from build123d import *

# Parameters (mm, degrees)
F0_R     = 25
F1_DEPTH = 5
F2_R     = 10
F3_DEPTH = 70
F4_R     = 19
F5_DEPTH = 5


with BuildPart() as f1:
    # F0 (on Front) → F1 (new body)
    with BuildSketch(Plane.XZ):
        Circle(F0_R)
    extrude(amount=F1_DEPTH)

    # F2 (on face) → F3 (join)
    with BuildSketch(Plane.XZ.offset(5)):
        Circle(F2_R)
    extrude(amount=F3_DEPTH)

    # F4 (on face) → F5 (join)
    with BuildSketch(Plane.XZ.offset(75)):
        Circle(F4_R)
    extrude(amount=F5_DEPTH)


solid = f1.part
Part model, mm, in its own coordinate system. A direction names the side the tool comes from. Coordinates: 2 decimals unless noted, no trailing zeros. Loops run counter-clockwise (first coordinate to the right, second up) from the corner with the lowest first, then second, coordinate; pieces in that order, holes last. Notation, with made-up numbers: (76, -15) - (86, -15) arc R8 cw to (86, -5) - close; hole circle Ø4 at (86.25, -37). An arc over 180 degrees is marked (long way). Write each question's results on one line, items separated by ' | '. Start each with the question number.
Q1. Slice it at D-D on y = -14. Give the cut face in (x, z).
Q2. Which spindle directions (+Z, -Z, +X, -X, +Y, -Y) get a long thin tool onto all of the face, cutting with end or side? Do faces 5 (the cylindrical face through (-2.17, -39.51, -9.76)), 6 (the cylindrical face through (8.767, -77.465, -16.856)), 7 (the cylindrical face through (23.846, -2.465, 7.509)). Say none if no direction does.
Q3. Drop flat-ended pins along their axis: pin 1 Ø3 at (y, z) = (-25.5, 5) entering from -X; pin 2 Ø12 at (x, y) = (11.5, -18) entering from +Z; pin 3 Ø5 at (y, z) = (-64, -9.5) entering from +X. Give the stop position or say it passes through.
Q4. Slice it at B-B on x = 0. Give the cut face in (y, z).
Q5. Two-plate mould, pull along Y, no slides. Class faces 1 (the flat face through (0, 0, 0)), 2 (the flat face through (0, -80, 0)), 3 (the flat face through (8, -75, -8)), 4 (the flat face through (0, -5, -11)): +Y half, -Y half, draft (parallel to the pull), parting line (faces both ways), or undercut.
Q6. Slice it at C-C on z = 13.5. Give the cut face in (x, y), and give its area (3 significant figures).
Q7. Probe line 1 along Y through (x, z) = (16.5, -2.5); line 2 along Y through (x, z) = (10, 22); line 3 along Z through (x, y) = (0.5, -36). List the from-to ranges inside material, lowest first.
Q8. Slice it at A-A on z = 0. Give the cut face in (x, y), and give its area (3 significant figures).
Answer:
1) outline: circle Ø20 at (0, 0)
2) face 5: none | face 6: -Y | face 7: +Y, -Y
3) pin 1: stops at x = -9.37 | pin 2: stops at z = 8.35 | pin 3: stops at x = 7.14
4) outline: (-80, -19) - (-75, -19) - (-75, -10) - (-5, -10) - (-5, -25) - (0, -25) - (0, 25) - (-5, 25) - (-5, 10) - (-75, 10) - (-75, 19) - (-80, 19) - close
5) face 1: +Y half | face 2: -Y half | face 3: undercut | face 4: undercut
6) outline: (-21.04, -5) - (21.04, -5) - (21.04, 0) - (-21.04, 0) - close; (-13.37, -80) - (13.37, -80) - (13.37, -75) - (-13.37, -75) - close | area: 344 mm2
7) line 1: y = -80 to -75, -5 to 0 | line 2: y = -5 to 0 | line 3: z = -9.99 to 9.99
8) outline: (-25, -5) - (-10, -5) - (-10, -75) - (-19, -75) - (-19, -80) - (19, -80) - (19, -75) - (10, -75) - (10, -5) - (25, -5) - (25, 0) - (-25, 0) - close | area: 1,840 mm2
